Drawing for the job (mm, zero at the part's lowest x, y, z). Give positions to 0.01 mm unless a question says otherwise; leave off trailing zeros. Order: outer loops, then holes, each group sorted by start corner. A loop starts at its lowest first (then second) coordinate and runs counter-clockwise, first axis right, second up. Notation, with made-up numbers: (63.5, 67.25) - (82.5, 67.25) arc R21 ccw to (82.5, 77.25) - close; hole circle Ø1 at (-32, 10). An arc over 180 degrees is marked (long way). Use a Markdown table: item, result.
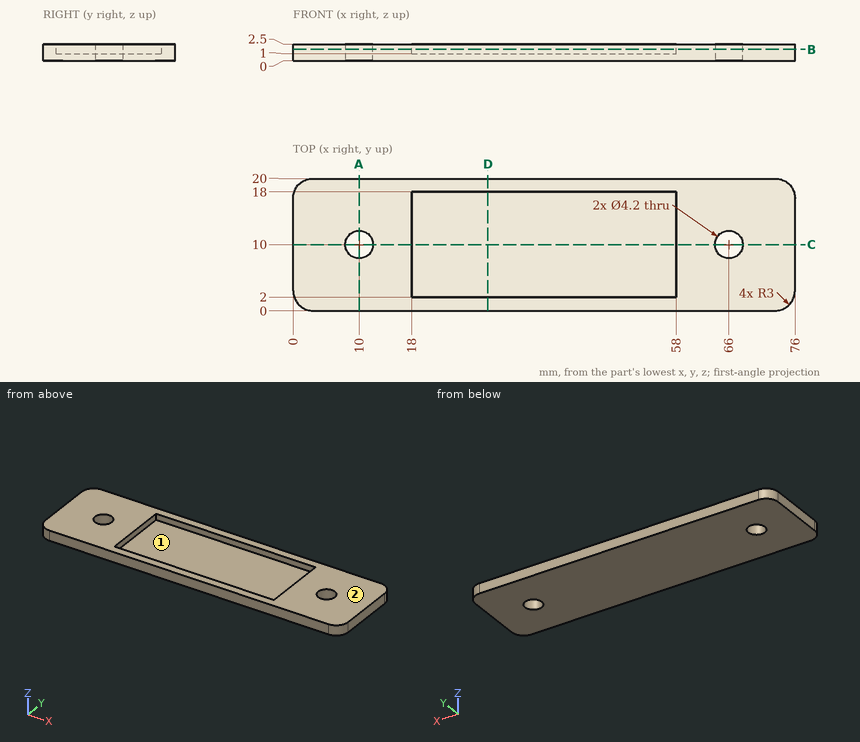
1) Slice it at C-C (y = 10). Write the cut outline in (x, z).
Computed:
| item | result |
|---|---|
| outline | (0, 0) - (7.9, 0) - (7.9, 2.5) - (0, 2.5) - close; (12.1, 0) - (63.9, 0) - (63.9, 2.5) - (58, 2.5) - (58, 1) - (18, 1) - (18, 2.5) - (12.1, 2.5) - close; (68.1, 0) - (76, 0) - (76, 2.5) - (68.1, 2.5) - close |
2) Slice it at B-B (z = 1.7). Write the cut outline in (x, y).
Computed:
| item | result |
|---|---|
| outline | (0, 3) arc R3 ccw to (3, 0) - (73, 0) arc R3 ccw to (76, 3) - (76, 17) arc R3 ccw to (73, 20) - (3, 20) arc R3 ccw to (0, 17) - close; hole circle Ø4.2 at (10, 10); hole (18, 2) - (58, 2) - (58, 18) - (18, 18) - close; hole circle Ø4.2 at (66, 10) |
3) Wall check: line 1 (X direction, y = 10, z = 1.9); line 2 (X direction, y = 10, z = 0.7); line 3 (Y direction, x = 10, z = 1.2). Give the ranges that are in metal, low to high. Write a range as from..to.
Computed:
| item | result |
|---|---|
| line 1 | x = 0..7.9, 12.1..18, 58..63.9, 68.1..76 |
| line 2 | x = 0..7.9, 12.1..63.9, 68.1..76 |
| line 3 | y = 0..7.9, 12.1..20 |
4) Pin check, flat tips, straight feed: P1, Ø3.5, axis at x = 10, y = 10, coming from the +Z side; P2, Ø5, axis at x = 36, y = 10.5, coming from the +Z side. Stop position of each tip, or through.
Computed:
| item | result |
|---|---|
| P1 | passes through |
| P2 | stops at z = 1 |
5) Slice it at A-A (x = 10). Write the cut outline in (y, z).
Computed:
| item | result |
|---|---|
| outline | (0, 0) - (7.9, 0) - (7.9, 2.5) - (0, 2.5) - close; (12.1, 0) - (20, 0) - (20, 2.5) - (12.1, 2.5) - close |
6) Two-plate mould, pull along Y, no slides. Class the marked faces 1 and 2: +Y half, -Y half, draft (parallel to the pull), parting line (faces both ways), or undercut.
Computed:
| item | result |
|---|---|
| face 1 | undercut |
| face 2 | draft |
7) Slice it at D-D (x = 29.5). Write the cut outline in (y, z), and give its area (3 significant figures).
Computed:
| item | result |
|---|---|
| outline | (0, 0) - (20, 0) - (20, 2.5) - (18, 2.5) - (18, 1) - (2, 1) - (2, 2.5) - (0, 2.5) - close |
| area | 26.0 mm² |
